The listing builds one solid part. Answer for the finished solid, in the listing's coordinates (mm). Round coordinates to 2 decimals unless told otherwise and drop trailing zeros. Write each loop counter-clockwise with the first axis right and the second up, starting at its lowest first coordinate (ties: lowest second). Pieces come first, ordered by that corner, then holes. Notation, with made-up numbers: M 35,28 L 78,28 A21 ccw 78,41 Z; hole C 5,14.5 d4. An arc over 180 degrees is marked long. One line per item, written item: value. Start each with the question number.
(1) Given P1, Ø4, axis at x = -11, y = -6.5, coming from the -Z side; P2, Ø2, axis at x = -18, y = -5, coming from the -Z side, each flat-ended and moving along its own axis, determine where each tip first touches the part or whether it passes through.
(2) Section C-C (y = -6) is taken. Determine the outline of the cut face in (x, z) (3 decimals), plus the area to 3 significant figures.
(3) Section B-B (z = 0) is taken. Determine the outline of the cut face in (x, y) (3 decimals).
(4) Section D-D (x = -24.5) is taken. Determine the outline of the cut face in (y, z), plus the area to 3 significant figures.
(5) Consider probe 1 along Z at (x, y) = (0, -3.25) (3 decimals); probe 2 along X at (y, z) = (-7.5, -4); probe 3 along X at (y, z) = (-4.25, -6) (3 decimals). Determine where each line is inside the solid, lowest interval first.
(6) For a pull along Z with two mould halves and no side action, classify faces 1 (the cylindrical face through (29.05, -3.94, -2.67)), 2 (the cylindrical face through (-36.107, -3.944, -27.686)), 3 (the flat face through (9, 0, 1)), 4 (the cylindrical face through (-27.184, -3.944, 0.307)) as released by +Z, released by -Z, zero draft, split by the parting line, or undercut.
(7) Section A-A (x = 0) is taken. Determine the outline of the cut face in (y, z) (3 decimals), plus the area to 3 significant figures.
```python
from build123d import *

# Parameters (mm, degrees)
F0_R     = 45.5
F2_DEPTH = 8
F1_R     = 3.175
F3_DEPTH = 8.001
F4_R     = 6.975
F5_DEPTH = 25


with BuildPart() as f2:
    # F0 (on Front) → F2 (new body)
    with BuildSketch(Plane.XZ):
        Circle(F0_R)
    extrude(amount=F2_DEPTH)

    # F1 (on Front) → F3 (cut, through all)
    with BuildSketch(Plane.XZ):
        Circle(F1_R)
    extrude(amount=F3_DEPTH, mode=Mode.SUBTRACT)

    # F4 (on Front) → F5 (cut)
    with BuildSketch(Plane.XZ):
        with Locations((-20.215824, 0)):
            Circle(F4_R)
        with Locations((22.608229, 0)):
            Circle(F4_R)
    extrude(amount=F5_DEPTH, mode=Mode.SUBTRACT)


solid = f2.part
```
Recorded:
1. P1: stops at z = -44.6
1. P2: stops at z = -42.2
2. outline: C 0,0 d91; hole C -20.216,0 d13.95; hole C 0,0 d6.35; hole C 22.608,0 d13.95
2. area: 6,170 mm2
3. outline: M -45.5,-8 L -27.191,-8 L -27.191,0 L -45.5,0 Z; M -13.241,-8 L -3.175,-8 L -3.175,0 L -13.241,0 Z; M 3.175,-8 L 15.633,-8 L 15.633,0 L 3.175,0 Z; M 29.583,-8 L 45.5,-8 L 45.5,0 L 29.583,0 Z
4. outline: M -8,-38.34 L 0,-38.34 L 0,-5.5 L -8,-5.5 Z; M -8,5.5 L 0,5.5 L 0,38.34 L -8,38.34 Z
4. area: 525 mm2
5. probe 1: z = -45.5 to -3.175, 3.175 to 45.5
5. probe 2: x = -45.32 to -25.93, -14.5 to 16.89, 28.32 to 45.32
5. probe 3: x = -45.103 to -23.773, -16.659 to 19.051, 26.165 to 45.103
6. face 1: undercut
6. face 2: split by the parting line
6. face 3: zero draft
6. face 4: undercut
7. outline: M -8,-45.5 L 0,-45.5 L 0,-3.175 L -8,-3.175 Z; M -8,3.175 L 0,3.175 L 0,45.5 L -8,45.5 Z
7. area: 677 mm2
